Print and shaded views of the part. All mm, measured from the part's lowest x, y and z. Coordinates: 2 decimals unless noted, no trailing zeros. Order: outer loops, then holes, each group sorted by start corner. A loop starts at its lowest first (then second) coordinate and runs counter-clockwise, first axis right, second up. Notation, with made-up numbers: (60.5, -34.5) -> (77.5, -34.5) arc R19 cw to (77.5, -11.5) -> close; hole circle Ø4 at (39.25, -7). An arc over 180 degrees is marked (long way). Write item = value, one per line. Start each with the question number.
Q1. Cut at C-C, the plane y = 3. List the corners of the cut face in (x, z).
Q2. Cut at A-A, the plane x = 6.25. List the corners of the cut face in (y, z), plus the area to 3 significant figures.
Q3. Mould opens along Z. For the marked faces 1, 2 and 3 say: +Z half, -Z half, draft (parallel to the pull), parting line (faces both ways), or undercut.
Q4. Cut at B-B, the plane z = 6. List the corners of the cut face in (x, y), plus the area to 3 significant figures.
Q5. Cut at D-D, the plane y = 1. List the corners of the cut face in (x, z), plus the area to 3 significant figures.
Q6. Flat gauge pin, fed straight in: pin 1 (5 mm diameter, centred on x = 6.25, z = 19.4, fed in from +Y). Where does the tip first touch, or does it go through?
Q7. Wall check: line 1 (Z direction, x = 6.25, y = 1.55); line 2 (X direction, y = 0.9, z = 19.4); line 3 (Z direction, x = 6.75, y = 0.7). Give the ranges that are in metal, low to high. Write a range as from..to.
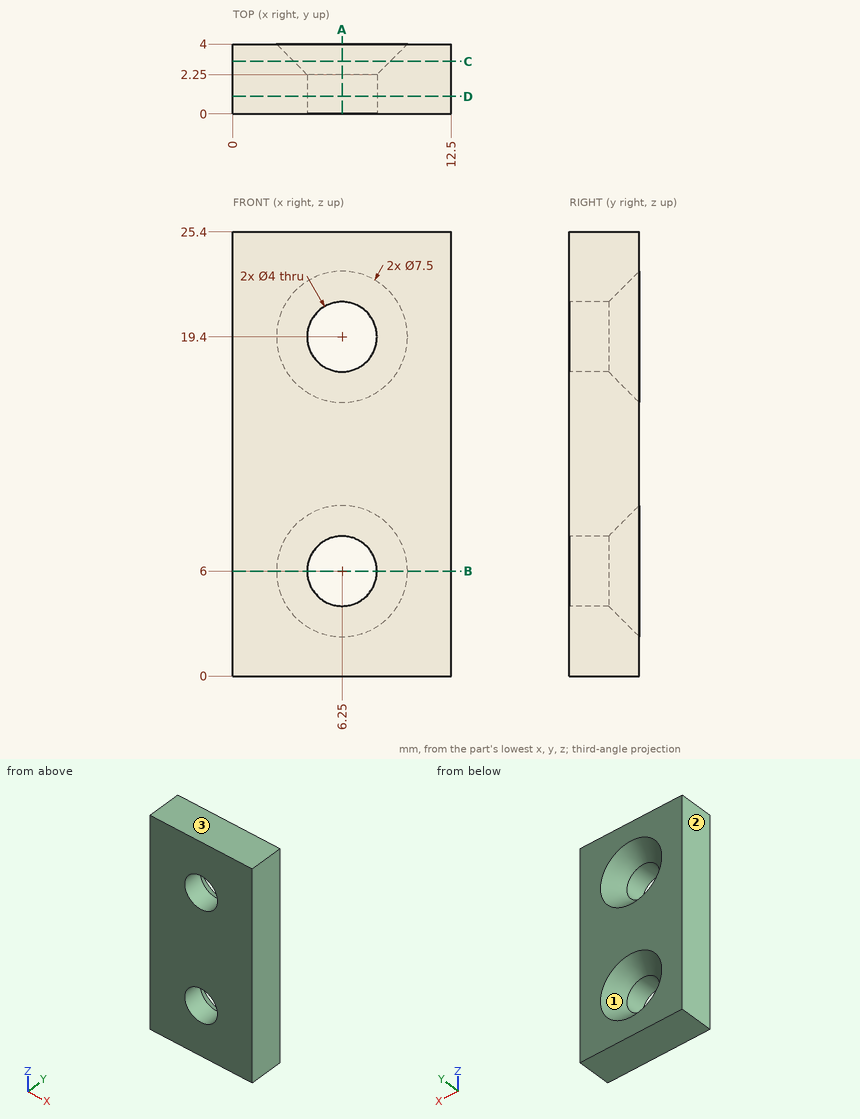
Here are the results:
q1.outline = (0, 0) -> (12.5, 0) -> (12.5, 25.4) -> (0, 25.4) -> close; hole circle Ø5.5 at (6.25, 6); hole circle Ø5.5 at (6.25, 19.4)
q2.outline = (0, 0) -> (4, 0) -> (4, 2.25) -> (2.25, 4) -> (0, 4) -> close; (0, 8) -> (2.25, 8) -> (4, 9.75) -> (4, 15.65) -> (2.25, 17.4) -> (0, 17.4) -> close; (0, 21.4) -> (2.25, 21.4) -> (4, 23.15) -> (4, 25.4) -> (0, 25.4) -> close
q2.area = 63.5 mm²
q3.face_1 = undercut
q3.face_2 = draft
q3.face_3 = +Z half
q4.outline = (0, 0) -> (4.25, 0) -> (4.25, 2.25) -> (2.5, 4) -> (0, 4) -> close; (8.25, 0) -> (12.5, 0) -> (12.5, 4) -> (10, 4) -> (8.25, 2.25) -> close
q4.area = 30.9 mm²
q5.outline = (0, 0) -> (12.5, 0) -> (12.5, 25.4) -> (0, 25.4) -> close; hole circle Ø4 at (6.25, 6); hole circle Ø4 at (6.25, 19.4)
q5.area = 292 mm²
q6.pin_1 = 2.75
q7.line_1 = 0..4, 8..17.4, 21.4..25.4
q7.line_2 = 0..4.25, 8.25..12.5
q7.line_3 = 0..4.06, 7.94..17.46, 21.34..25.4
